Here's how the part is built. I have some questions about the finished solid (model axes, mm). A direction names the side the tool comes from. Round coordinates to 2 decimals unless told otherwise and drop trailing zeros. Loops run counter-clockwise (first coordinate to the right, second up) from the corner with the lowest first, then second, coordinate; pieces in that order, holes last. Notation, with made-up numbers: M 76.5,-29 L 90.5,-29 A15 ccw 90.5,-5 Z; hole C 88.5,56.5 d6. An arc over 180 degrees is marked long. Write each question's results on one line, items separated by ' | '. Start each with the question number.
```python
from build123d import *

# Parameters (mm, degrees)
F0_W     = 500
F0_H     = 190
F1_DEPTH = 20
F2_W     = 500
F2_H     = 300
F3_DEPTH = 20


# Not quite as in the source:
# - the program builds the solid bodies; features that only make, move or delete a surface that nothing else refers to are left out


with BuildPart() as f1:
    # F0 (on Top) → F1 (new body)
    with BuildSketch(Plane.XY):
        with Locations((0, -95)):
            Rectangle(F0_W, F0_H)
    extrude(amount=-F1_DEPTH)

    # F2 (on Front) → F3 (join)
    with BuildSketch(Plane.XZ):
        with Locations((0, -150)):
            Rectangle(F2_W, F2_H)
    extrude(amount=F3_DEPTH)


solid = f1.part
```
1. For pin 1 (1.5 mm diameter, centred on x = 183, z = -253.5, fed in from -Y); pin 2 (1.5 mm diameter, centred on x = -139.5, y = -31.5, fed in from +Z), each with a flat end and sliding along its axis, tell me the tip position at first contact or that it passes through.
2. Which directions (+Z, -Z, +X, -X, +Y, -Y) give clear straight access to the entire face, cutting with the end or side of a thin tool? Please do faces 1 (the face through (-3, -20, -158)), 2 (the face through (-250, -17, -95)).
3. I want a section at B-B on z = -138. List the corners of the cut face in (x, y) for me.
4. I need wall thicknesses on line 1 along Z through (x, y) = (27, -53.5). Which ranges of the line are inside material? Lowest first, please.
5. I want a section at A-A on x = -146. List the corners of the cut face in (y, z) for me, plus the area to 3 significant figures.
Outcome:
1) pin 1: y = -20 | pin 2: z = 0
2) face 1: -Z, +X, -X, -Y | face 2: +Z, -Z, -X, +Y, -Y
3) outline: M -250,-20 L 250,-20 L 250,0 L -250,0 Z
4) line 1: -20 to 0
5) outline: M -190,-20 L -20,-20 L -20,-300 L 0,-300 L 0,0 L -190,0 Z | area: 9,400 mm2
